```python
from build123d import *

# Parameters (mm, degrees)
CROQUIS1_R              = 4
CROQUIS1_R_2            = 1.1
SALIENTE_EXTRUIR1_DEPTH = 2.5
CROQUIS2_W              = 13.1
CROQUIS2_H              = 2
CORTAR_EXTRUIR1_DEPTH   = 15
CORTAR_EXTRUIR2_REACH   = 30.748
CROQUIS3_R              = 10.7
REDONDEO1_R             = 1.6


with BuildPart() as part:
    # Croquis1 → Saliente-Extruir1 (new, symmetric)
    with BuildSketch(Plane(origin=(0, 0, 0), x_dir=(1, 0, 0), z_dir=(0, 1, 0))):
        with BuildLine():
            Line((-25.76696336, 10.35), (-7.009101226, 10.35))
            ThreePointArc((-7.009101226, 10.35), (12.5, 0), (-7.009101226, -10.35))
            Line((-7.009101226, -10.35), (-25.76696336, -10.35))
            Line((-25.76696336, -10.35), (-25.76696336, 10.35))
        make_face()
        with Locations(Location((0, 0, 0), (0, 0, 270))):
            Circle(CROQUIS1_R, mode=Mode.SUBTRACT)
        with Locations(Location((0, 7, 0), (0, 0, 270))):
            Circle(CROQUIS1_R_2, mode=Mode.SUBTRACT)
        with Locations(Location((0, -7, 0), (0, 0, 90))):
            Circle(CROQUIS1_R_2, mode=Mode.SUBTRACT)
    extrude(amount=SALIENTE_EXTRUIR1_DEPTH, both=True)

    # Croquis2 → Cortar-Extruir1 (cut)
    with BuildSketch(Plane.ZY.offset(25.76696336)):
        Rectangle(CROQUIS2_W, CROQUIS2_H)
    extrude(amount=-CORTAR_EXTRUIR1_DEPTH, mode=Mode.SUBTRACT)

    # Croquis3 → Cortar-Extruir2 (cut, up to next)
    with BuildSketch(Plane(origin=(0, 0, 0), x_dir=(1, 0, 0), z_dir=(0, 1, 0)), mode=Mode.PRIVATE) as cortar_extruir2_sk1:
        with Locations(Location((0, 0, 0), (0, 0, 270))):
            Circle(CROQUIS3_R)
    cortar_extruir2_tool1 = extrude(cortar_extruir2_sk1.sketch, amount=-CORTAR_EXTRUIR2_REACH, mode=Mode.PRIVATE) & part.part
    add(cortar_extruir2_tool1.solids().sort_by_distance((0, 0, 0))[0], mode=Mode.SUBTRACT)

    # Redondeo1
    redondeo1_edges = [part.edges().sort_by_distance(p)[0] for p in [
        (12.5, 2.5, 0),
        (-16.388032293, 2.5, -10.35),
        (-16.388032293, -2.5, -10.35),
        (12.5, -2.5, 0),
        (-16.388032293, -2.5, 10.35),
        (-16.388032293, 2.5, 10.35),
        (-7.009101226, 0, -10.35),
        (-7.009101226, 0, 10.35),
    ]]
    fillet(redondeo1_edges, radius=REDONDEO1_R)


solid = part.part
```
Geometry check sheet. Reference: the model listing, model coordinates, mm. A direction names the side the tool comes from. Round coordinates to 2 decimals unless told otherwise and drop trailing zeros. Loops run counter-clockwise (first coordinate to the right, second up) from the corner with the lowest first, then second, coordinate; pieces in that order, holes last. Notation, with made-up numbers: (-21.5, 57) -> (21.5, 57) arc R36 cw to (21.5, 95) -> close; hole circle Ø8 at (20.5, 32.5). An arc over 180 degrees is marked (long way). Use a Markdown table: item, result.
(1) Sectioned sample at B-B (x = 0). Give the number of separate pieces and of enclosed holes in the cut face, then the cut area to 3 significant figures.
Calculated:
| item | result |
|---|---|
| separate pieces | 4 |
| enclosed holes | 0 |
| area | 38.3 mm² |
(2) Set-up check for faces 1 (the cylindrical face through (-16.75, -2.04, 9.87)), 2 (the cylindrical face through (-16.5, -2.02, -9.89)), 3 (the cylindrical face through (-10.446, -1.232, -2.32)), 4 (the flat face through (-18, 0, -6.55)): record each of +Z, -Z, +X, -X, +Y, -Y from which the full face is reachable in a straight line by a thin tool's end or side.
Calculated:
| item | result |
|---|---|
| face 1 | +Z, -X, -Y |
| face 2 | -Z, -X, -Y |
| face 3 | -Y |
| face 4 | -X |
(3) Sectioned sample at A-A (z = 0). Enter the section's corners in (x, y).
Calculated:
| item | result |
|---|---|
| outline | (-25.77, -2.5) -> (-10.7, -2.5) -> (-10.7, 0) -> (-4, 0) -> (-4, 2.5) -> (-25.77, 2.5) -> (-25.77, 1) -> (-10.77, 1) -> (-10.77, -1) -> (-25.77, -1) -> close; (4, 0) -> (10.7, 0) -> (10.7, -2.5) -> (10.9, -2.5) arc R1.6 ccw to (12.5, -0.9) -> (12.5, 0.9) arc R1.6 ccw to (10.9, 2.5) -> (4, 2.5) -> close |
(4) Sectioned sample at C-C (y = 1.75). Enter the section's corners in (x, z).
Calculated:
| item | result |
|---|---|
| outline | (-25.77, -10.11) -> (-7.48, -10.11) arc R1.84 cw to (-6.5, -10.39) arc R12.26 ccw (long way) to (-6.5, 10.39) arc R1.84 cw to (-7.48, 10.11) -> (-25.77, 10.11) -> close; hole circle Ø8 at (0, 0); hole circle Ø2.2 at (0, -7); hole circle Ø2.2 at (0, 7) |
(5) Mould release check, pull along Y, two halves, no side actions. Record for faces 5 (the cylindrical face through (-7.036, -0.013, 10.414)), 6 (the flat face through (-10.767, 0.2, -0.1)), 7 (the flat face through (-7, 2.5, 0)): released by +Y, released by -Y, zero draft, split by the parting line, or undercut.
Calculated:
| item | result |
|---|---|
| face 5 | zero draft |
| face 6 | undercut |
| face 7 | released by +Y |
(6) Sectioned sample at D-D (y = -1.9). Enter the section's corners in (x, z), then the cut area to 3 significant figures.
Calculated:
| item | result |
|---|---|
| outline | (-25.77, -10) -> (-7.48, -10) arc R1.95 cw to (-6.45, -10.3) arc R12.15 ccw (long way) to (-6.45, 10.3) arc R1.95 cw to (-7.48, 10) -> (-25.77, 10) -> close; hole circle Ø21.4 at (0, 0) |
| area | 408 mm² |
(7) Scan lines: probe 1 along Z at (x, y) = (-11, 0.3); probe 2 along Y at (x, z) = (-17.5, -6.5); probe 3 along X at (y, z) = (0.6, 0). Record each from-to range of solid material in increasing order.
Calculated:
| item | result |
|---|---|
| probe 1 | -10.35 to -6.55, 6.55 to 10.35 |
| probe 2 | -2.5 to -1, 1 to 2.5 |
| probe 3 | -10.77 to -4, 4 to 12.5 |
(8) Go/stop test with flat-tipped pins: P1, Ø0.6, axis at x = -18, y = 0.5, coming from the -Z side; P2, Ø1.8, axis at x = 0, z = -7, coming from the -Y side; P3, Ø2, axis at x = 8, y = 1, coming from the -Z side; P4, Ø2, axis at x = -20.5, y = 0.5, coming from the +Z side. Record where each tip stops, or that it passes through.
Calculated:
| item | result |
|---|---|
| P1 | z = -10.35 |
| P2 | through |
| P3 | z = -10.35 |
| P4 | z = 10.35 |
